Source: CAD feature listing. Evaluate the final solid. Frame: model axes, mm. Face numbers are marked on the shaded views. A direction names the side the tool comes from. Coordinates: 2 decimals unless noted, no trailing zeros. Order: outer loops, then holes, each group sorted by start corner. A loop starts at its lowest first (then second) coordinate and runs counter-clockwise, first axis right, second up.
Item 1: Section B-B on z = 23.31. Return the cut outline in (x, y).
Item 2: Section C-C on y = -8. State how many separate pieces and enclosed holes the cut face has, then the cut area to 3 significant figures.
Item 3: Ray query, line 1 (Z direction, x = 17, y = -8); line 2 (X direction, y = -1.75, z = 19); line 3 (X direction, y = -13.5, z = 7.5). Return the intervals inside material, ascending.
Item 4: Section A-A on z = 4. Return the cut outline in (x, y).
Item 5: Section D-D on x = 48. Return the cut outline in (y, z), then the cut area to 3 significant figures.
Item 6: Contact query for flat-ended pins moving along their axis: P1, Ø2, axis at y = -3, z = 11.5, coming from the -X side; P2, Ø4, axis at x = 50, y = -7, coming from the +Z side; P3, Ø1, axis at y = -5, z = 16.5, coming from the +X side. Output: stop coordinate, or through.
Item 7: Reachability of the marked faces 5, 6, 7 and 8 from +Z, -Z, +X, -X, +Y, -Y: full face, straight path, thin tool, end or side. Return the list, or none.
Item 8: Mould query, pull axis Y, two halves, no side actions, for the marked faces 1, 2, 3 and 4. Classes: released by +Y, released by -Y, zero draft, split by the parting line, or undercut.
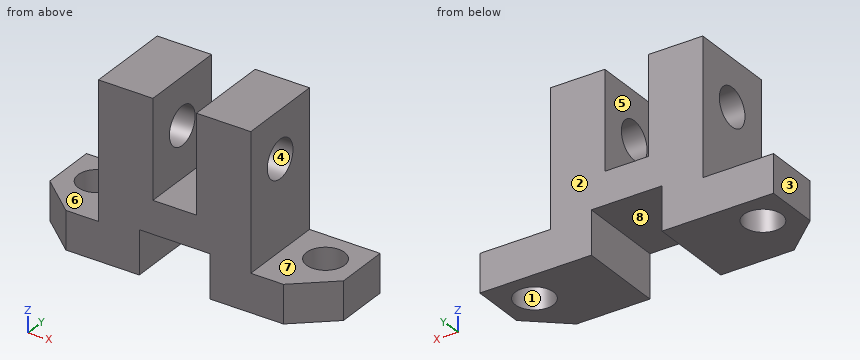
from build123d import *

# Parameters (mm, degrees)
PAD_DEPTH       = 32
SKETCH001_W     = 13
SKETCH001_H     = 16
POCKET_DEPTH    = 8
POCKET001_DEPTH = 25
POCKET002_DEPTH = 25
SKETCH004_W     = 8
SKETCH004_H     = 16
POCKET003_DEPTH = 18
SKETCH005_R     = 3.5
POCKET004_DEPTH = 8
SKETCH006_R     = 3.5
POCKET005_DEPTH = 30


with BuildPart() as part:
    # Sketch → Pad (new body)
    with BuildSketch(Plane.XY):
        Polygon((0, 0), (0, -10), (7, -16), (47, -16), (54, -10), (54, 0), align=None)
    extrude(amount=PAD_DEPTH)

    # Sketch001 (on Face7 of Pad) → Pocket (cut)
    with BuildSketch(Plane(origin=(0, 0, 0), x_dir=(1, 0, 0), z_dir=(0, 0, -1))):
        with Locations((27, 8)):
            Rectangle(SKETCH001_W, SKETCH001_H)
    extrude(amount=-POCKET_DEPTH, mode=Mode.SUBTRACT)

    # Sketch002 (on Face5 of Pocket) → Pocket001 (cut)
    with BuildSketch(Plane.XY.offset(32)):
        Polygon((0, 0), (0, -10), (7, -16), (13, -16), (13, 0), align=None)
    extrude(amount=-POCKET001_DEPTH, mode=Mode.SUBTRACT)

    # Sketch003 (on Face12 of Pocket001) → Pocket002 (cut)
    with BuildSketch(Plane.XY.offset(32)):
        Polygon((54, 0), (41, 0), (41, -16), (47, -16), (54, -10), align=None)
    extrude(amount=-POCKET002_DEPTH, mode=Mode.SUBTRACT)

    # Sketch004 (on Face12 of Pocket002) → Pocket003 (cut)
    with BuildSketch(Plane.XY.offset(32)):
        with Locations((27, -8)):
            Rectangle(SKETCH004_W, SKETCH004_H)
    extrude(amount=-POCKET003_DEPTH, mode=Mode.SUBTRACT)

    # Sketch005 (on Face4 of Pocket003) → Pocket004 (cut)
    with BuildSketch(Plane.XY.offset(7)):
        with Locations((6, -6)):
            Circle(SKETCH005_R)
        with Locations((48, -6)):
            Circle(SKETCH005_R)
    extrude(amount=-POCKET004_DEPTH, mode=Mode.SUBTRACT)

    # Sketch006 (on Face9 of Pocket004) → Pocket005 (cut)
    with BuildSketch(Plane(origin=(13, 0, 0), x_dir=(0, -1, 0), z_dir=(-1, 0, 0))):
        with Locations((8, 23.31)):
            Circle(SKETCH006_R)
    extrude(amount=-POCKET005_DEPTH, mode=Mode.SUBTRACT)


solid = part.part
Answer list:
1. outline: (13, -16) - (23, -16) - (23, -11.5) - (13, -11.5) - close; (13, -4.5) - (23, -4.5) - (23, 0) - (13, 0) - close; (31, -16) - (41, -16) - (41, -11.5) - (31, -11.5) - close; (31, -4.5) - (41, -4.5) - (41, 0) - (31, 0) - close
2. separate pieces: 5
2. enclosed holes: 0
2. area: 610 mm2
3. line 1: z = 0 to 19.81, 26.81 to 32
3. line 2: x = 13 to 23, 31 to 41
3. line 3: x = 13 to 20.5, 33.5 to 41
4. outline: (0, -10) - (7, -16) - (20.5, -16) - (20.5, 0) - (0, 0) - close; (33.5, -16) - (47, -16) - (54, -10) - (54, 0) - (33.5, 0) - close; hole circle Ø7 at (6, -6); hole circle Ø7 at (48, -6)
5. outline: (-15.14, 0) - (-9.5, 0) - (-9.5, 7) - (-15.14, 7) - close; (-2.5, 0) - (0, 0) - (0, 7) - (-2.5, 7) - close
5. area: 57.0 mm2
6. P1: stops at x = 13
6. P2: stops at z = 7
6. P3: stops at x = 41
7. face 5: +Z, +Y, -Y
7. face 6: +Z, -X, +Y, -Y
7. face 7: +Z, +X, +Y, -Y
7. face 8: -Z, +Y, -Y
8. face 1: undercut
8. face 2: released by +Y
8. face 3: zero draft
8. face 4: undercut
